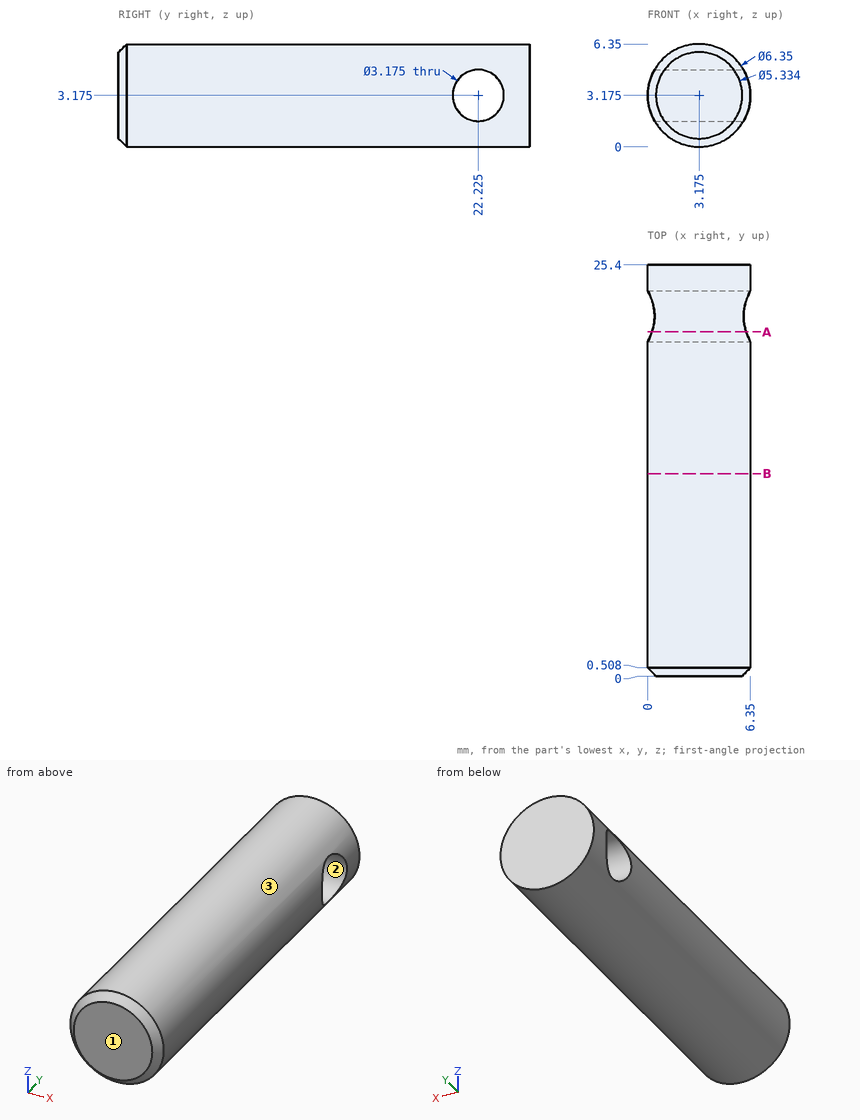
The drawing under review shows one solid part. Ordinate dimensions are in mm from its lowest x, y, z. Round coordinates to 2 decimals unless told otherwise and drop trailing zeros. Write each loop counter-clockwise with the first axis right and the second up, starting at its lowest first coordinate (ties: lowest second). Pieces come first, ordered by that corner, then holes. Notation, with made-up numbers: (-23.75, 54) -> (21.25, 54) arc R10 ccw to (21.25, 68) -> close; hole circle Ø10 at (4.5, 48). An arc over 180 degrees is marked (long way). One line per question, with ' | ' between items. Start each with the question number.
(1) Mouldability with a two-part tool opening along Z and no side actions: class the marked faces 1, 2 and 3 as released by +Z, released by -Z, zero draft, split by the parting line, or undercut.
(2) Add section B-B, the plane y = 12.5. Write out the cut boundary in (x, z) (3 decimals).
(3) For line 1 along Y through (x, z) = (3.75, 3.25); line 2 along X through (y, z) = (6.5, 3.25); line 3 along Z through (x, y) = (4.5, 22.25), list the stretches that pass through material, from the lowest coordinate up. Write a range as from..to.
(4) Insertion check: P1, Ø1.5, axis at x = 1.5, y = 21.5, coming from the +Z side. The pin has a flat end and moves straight along its axis. Give the tip position at first contact, or say it passes through.
(5) Add section A-A, the plane y = 21.25. Write out the cut boundary in (x, z) (3 decimals).
Answer list:
1) face 1: zero draft | face 2: undercut | face 3: split by the parting line
2) outline: circle Ø6.35 at (3.175, 3.175)
3) line 1: 0..20.64, 23.81..25.4 | line 2: 0..6.35 | line 3: 0.29..1.59, 4.76..6.06
4) P1: z = 6.21
5) outline: (0.258, 1.922) arc R3.175 ccw to (6.092, 1.922) -> close; (0.258, 4.428) -> (6.092, 4.428) arc R3.175 ccw to start
